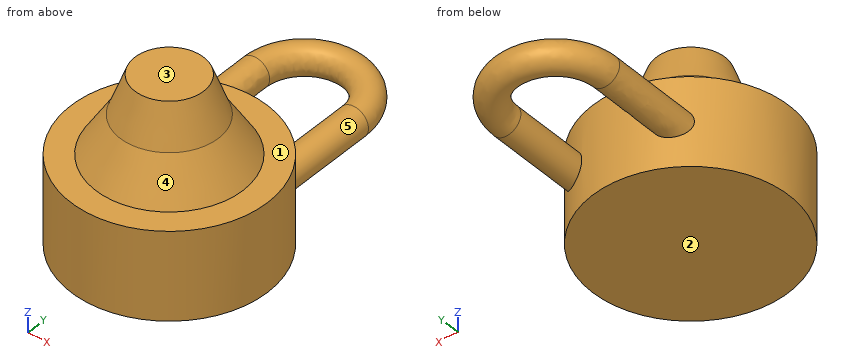
Autodesk Inventor part; units mm, degrees
ref_plane "Work Plane1" through (0, 0, 13) normal (0, 0, 1) x (1, 0, 0)
ref_plane "Work Plane2" through (0, 0, 17) normal (0, 0, 1) x (1, 0, 0)
ref_plane "Work Plane3" through (0, 0, 4.5) normal (0, 0, 1) x (1, 0, 0)
sketch "Sketch1" plane through (0, 0, 0) normal (0, 0, 1) x (1, 0, 0)
  circle A0 centre (0, 0) radius 10
  dimension "d0" = 20
extrude "Extrusion1" add sketch "Sketch1" along normal blind 9
sketch "Sketch2" plane through (0, 0, 9) normal (0, 0, 1) x (1, 0, 0)
  circle A0 centre (0, 0) radius 7.5
  dimension "d3" = 15
ref_plane "Work Plane1" through (0, 0, 13) normal (0, 0, 1) x (1, 0, 0)
sketch "Sketch3" plane through (0, 0, 13) normal (0, 0, 1) x (1, 0, 0)
  circle A0 centre (0, 0) radius 5
  dimension "d5" = 10
loft "Loft1" add profiles "Sketch2", "Sketch3"
sketch "Sketch4" plane through (0, 0, 13) normal (0, 0, 1) x (1, 0, 0)
  circle A0 centre (0, 0) radius 5
  dimension "d10" = 10
ref_plane "Work Plane2" through (0, 0, 17) normal (0, 0, 1) x (1, 0, 0)
sketch "Sketch5" plane through (0, 0, 17) normal (0, 0, 1) x (1, 0, 0)
  circle A0 centre (0, 0) radius 3.5
  dimension "d12" = 7
loft "Loft2" add profiles "Sketch5" section 1 edges at (-5, 0, 13)
ref_plane "Work Plane3" through (0, 0, 4.5) normal (0, 0, 1) x (1, 0, 0)
sketch "Sketch6" plane through (0, 0, 4.5) normal (0, 0, 1) x (1, 0, 0)
  arc A0 (5, 17) -> (-5.0779, 16.9998) centre (-0.0389, 17) ccw
  line L0 (5, 17) -> (5, 0)
  circle A1 centre (0, 0) radius 5
  line L1 (5, 17) -> (22, 17) construction
  line L2 (-5.0779, 16.9998) -> (-5, 0)
  line L3 (0, 0) -> (0, 5)
  dimension "d20" = 17
  dimension "d21" = 90
  dimension "d22" = 17
ref_plane "Work Plane4" through (5, 0, 4.5) normal (0, -1, 0) x (1, 0, 0)
sketch "Sketch7" plane through (5, 0, 4.5) normal (0, -1, 0) x (1, 0, 0)
  circle A0 centre (0, 0) radius 1.5
  point P0 (-5, -4.5)
  dimension "d23" = 3
sweep "Sweep1" add profiles "Sketch7" path "Sketch6" path curves L0 A0 L2
properties part number "padlock"
Work out the finished part from the listing and answer in its coordinate system (mm). Face numbers are marked on the shaded views. A direction names the side the tool comes from. Give positions to 0.01 mm unless a question says otherwise; leave off trailing zeros. Write each loop counter-clockwise with the first axis right and the second up, starting at its lowest first coordinate (ties: lowest second). Pieces come first, ordered by that corner, then holes. Notation, with made-up numbers: (-5, -21.75) -> (51, -21.75) arc R10 cw to (51, -9.75) -> close; hole circle Ø8 at (-34.75, 13). An arc over 180 degrees is marked (long way). Write item = value, one per line.
Q1. Flat-ended cylindrical pins translate along their axes: pin 1 Ø1 at (y, z) = (3, 8.5) entering from +X; pin 2 Ø8 at (x, z) = (7, 2) entering from +Y; pin 3 Ø1.5 at (x, z) = (-4, 11.5) entering from -Y. Find the tip coordinate at first contact, or state that the pin passes through.
Computed values:
pin_1 = 9.68
pin_2 = 22.37
pin_3 = -5.22
Q2. A tool of negligible diameter and unlimited length cuts with its end or side. For the marked faces 1 and 2, from which of +Z, -Z, +X, -X, +Y, -Y can it reach the whole face along a straight path? Write none if from no direction.
Computed values:
face_1 = +Z
face_2 = -Z, +X, -X, +Y, -Y
Q3. For a pull along X with two mould halves and no side action, classify the marked faces 3, 4 and 5 as pulls with the +X half, pulls with the -X half, needs draft (parallel to the pull), parting line crosses it, or undercut.
Computed values:
face_3 = needs draft
face_4 = parting line crosses it
face_5 = undercut
Q4. Section B-B on x = 8.5 is taken. Determine the outline of the cut face in (y, z).
Computed values:
outline = (-5.27, 0) -> (5.27, 0) -> (5.27, 9) -> (-5.27, 9) -> close
Q5. Consider line 1 along Z through (x, y) = (-7.25, -5.5); line 2 along X through (y, z) = (18, 4.5); line 3 along Y through (x, z) = (-0.5, 5.5). Determine where each line is inside the solid, lowest interval first.
Computed values:
line_1 = 0 to 9
line_2 = -6.5 to -3.43, 3.36 to 6.42
line_3 = -9.99 to 9.99, 20.89 to 23.14
Q6. Section A-A on z = 2.5 is taken. Determine the outline of the cut face in (x, y).
Computed values:
outline = circle Ø20 at (0, 0)
